```python
from build123d import *

# Parameters (mm, degrees)
SKETCH1_R           = 1.65
SKETCH1_W           = 3
SKETCH1_H           = 20
SKETCH1_W_2         = 24
SKETCH1_H_2         = 22.230872535
BOSS_EXTRUDE2_DEPTH = 3
SKETCH3_W           = 102.87568526
SKETCH3_H           = 126.113289936
CUT_EXTRUDE1_DEPTH  = 10


with BuildPart() as part:
    # Sketch1 → Boss-Extrude2 (new body)
    with BuildSketch(Plane.XY):
        Polygon((-59.447183423, 47.780041818), (-49.447183423, 57.780041818), (20.552816577, 57.780041818), (30.552816577, 47.780041818), (30.552816577, -0.7691812), (26.052816577, -5.2691812), (25.552816577, -5.2691812), (25.552816577, -50.590735163), (26.052816577, -50.590735163), (30.552816577, -55.090735163), (30.552816577, -103.639958182), (20.552816577, -113.639958182), (-49.447183423, -113.639958182), (-59.447183423, -103.639958182), (-59.447183423, -55.090735163), (-54.947183423, -50.590735163), (-54.447183423, -50.590735163), (-54.447183423, -5.2691812), (-54.947183423, -5.2691812), (-59.447183423, -0.7691812), align=None)
        with Locations((-39.447183423, 52.780041818)):
            Circle(SKETCH1_R, mode=Mode.SUBTRACT)
        with Locations((10.552816577, 52.780041818)):
            Circle(SKETCH1_R, mode=Mode.SUBTRACT)
        with Locations(Location((10.552816577, -108.639958182, 0), (0, 0, 180))):
            Circle(SKETCH1_R, mode=Mode.SUBTRACT)
        with Locations(Location((-39.447183423, -108.639958182, 0), (0, 0, 180))):
            Circle(SKETCH1_R, mode=Mode.SUBTRACT)
        with Locations((10.552816577, -62.748057161)):
            Circle(SKETCH1_R, mode=Mode.SUBTRACT)
        with Locations(Location((-39.447183423, -62.748057161, 0), (0, 0, 180))):
            Circle(SKETCH1_R, mode=Mode.SUBTRACT)
        with Locations((-27.947183423, 11.175041818)):
            Rectangle(SKETCH1_W, SKETCH1_H, mode=Mode.SUBTRACT)
        with Locations((-0.947183423, 11.175041818)):
            Rectangle(SKETCH1_W, SKETCH1_H, mode=Mode.SUBTRACT)
        with Locations((-14.447183423, -27.929958181)):
            Rectangle(SKETCH1_W_2, SKETCH1_H_2, mode=Mode.SUBTRACT)
    extrude(amount=BOSS_EXTRUDE2_DEPTH)

    # Sketch3 → Cut-Extrude1 (cut)
    with BuildSketch(Plane.XY.offset(3)):
        with Locations((-8.901321225, 12.465909805)):
            Rectangle(SKETCH3_W, SKETCH3_H)
    extrude(amount=-CUT_EXTRUDE1_DEPTH, mode=Mode.SUBTRACT)


solid = part.part
```
Design review of the part built by this model. Coordinates are the model's own, in mm. Round coordinates to 2 decimals unless told otherwise and drop trailing zeros. Order: outer loops, then holes, each group sorted by start corner. A loop starts at its lowest first (then second) coordinate and runs counter-clockwise, first axis right, second up. Notation, with made-up numbers: (87.5, 12.25) - (129.5, 12.25) arc R12 cw to (129.5, 26.25) - close; hole circle Ø11 at (23.25, 73). An arc over 180 degrees is marked (long way). Return JSON: item names as keys, results as strings.
Q1. Consider section A-A on z = 1.85. Write out the cut boundary in (x, y).
Computed values:
{"outline": "(-59.45, -103.64) - (-49.45, -113.64) - (20.55, -113.64) - (30.55, -103.64) - (30.55, -55.09) - (26.05, -50.59) - (-54.95, -50.59) - (-59.45, -55.09) - close; hole circle Ø3.3 at (-39.45, -108.64); hole circle Ø3.3 at (-39.45, -62.75); hole circle Ø3.3 at (10.55, -108.64); hole circle Ø3.3 at (10.55, -62.75)"}
Q2. For pin 1 Ø1.5 at (x, y) = (-18.5, -90) entering from -Z, flat-tipped, find the tip position at first contact; note if it passes through.
Computed values:
{"pin 1": "stops at z = 0"}
Q3. Wall thickness on L1, parallel to X at y = -108, z = 2.35; L2, parallel to X at y = -108.5, z = 1: over which ranges is each line inside the solid? List them lowest first. Write a range as [from, to].
Computed values:
{"L1": "x = [-55.09, -40.97], [-37.93, 9.03], [12.07, 26.19]", "L2": "x = [-54.59, -41.09], [-37.8, 8.91], [12.2, 25.69]"}
Q4. The part is to be moulded in two halves that separate along Y. For faces 1 (the flat face through (-54.377, -108.71, 1.479)), 2 (the flat face through (-59.447, -80, 1)), 3 (the cylindrical face through (11.314, -64.212, 1.479)), say which applies: pulls with the +Y half, pulls with the -Y half, needs draft (parallel to the pull), parting line crosses it, or undercut.
Computed values:
{"face 1": "pulls with the -Y half", "face 2": "needs draft", "face 3": "undercut"}
